Geometry: see drawing. Coordinates: mm, zero at the bounding-box minimum. A direction names the side the tool comes from. Round coordinates to 2 decimals unless told otherwise and drop trailing zeros. Loops run counter-clockwise (first coordinate to the right, second up) from the corner with the lowest first, then second, coordinate; pieces in that order, holes last. Notation, with made-up numbers: (51.25, 69.25) -> (86.25, 69.25) arc R31 cw to (86.25, 105.25) -> close; hole circle Ø9 at (84.25, 33.5). An arc over 180 degrees is marked (long way). Write item = value, one per line.
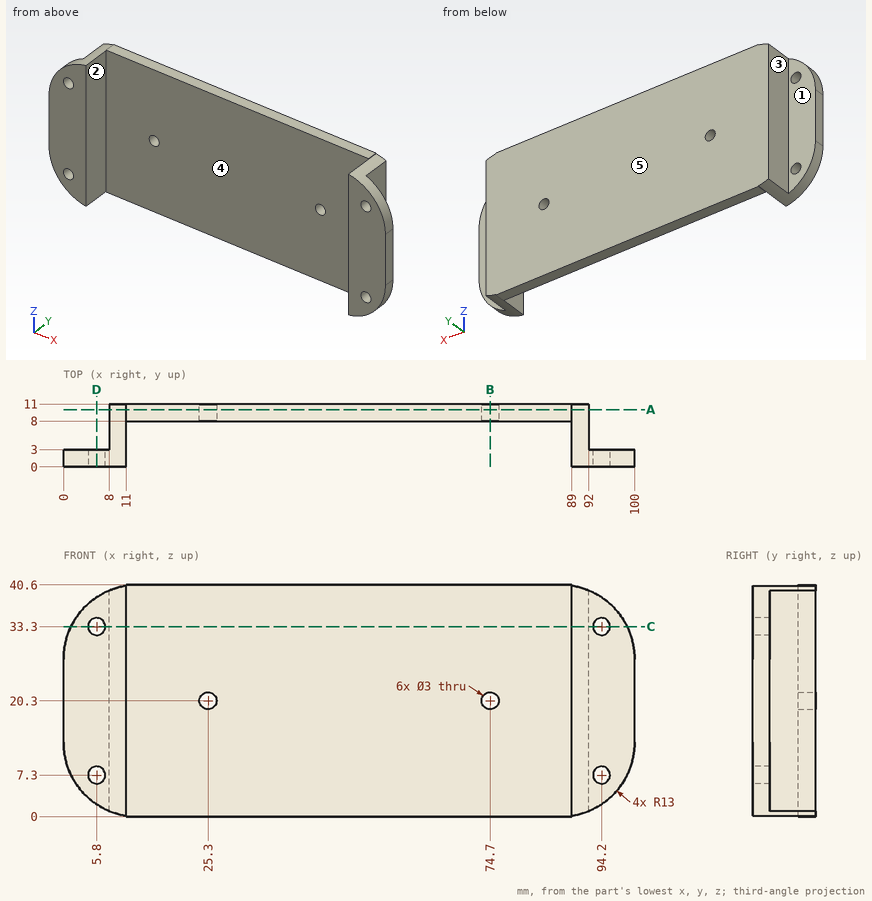
1. Section query C-C (z = 33.3). Return the cut outline in (x, y).
Evaluation:
outline = (1.32, 0) -> (4.3, 0) -> (4.3, 3) -> (1.32, 3) -> close; (7.3, 0) -> (11, 0) -> (11, 8) -> (89, 8) -> (89, 0) -> (92.7, 0) -> (92.7, 3) -> (92, 3) -> (92, 11) -> (8, 11) -> (8, 3) -> (7.3, 3) -> close; (95.7, 0) -> (98.68, 0) -> (98.68, 3) -> (95.7, 3) -> close
2. Section query B-B (x = 74.7). Return the cut outline in (y, z).
Evaluation:
outline = (8, 0) -> (11, 0) -> (11, 18.8) -> (8, 18.8) -> close; (8, 21.8) -> (11, 21.8) -> (11, 40.6) -> (8, 40.6) -> close
3. Contact query for flat-ended pins moving along their axis: pin 1 Ø4 at (x, z) = (5.5, 25.5) entering from +Y; pin 2 Ø2.5 at (y, z) = (6, 27.5) entering from +X; pin 3 Ø2 at (y, z) = (8.5, 13.5) entering from -X. Output: stop coordinate, or through.
Evaluation:
pin_1 = 3
pin_2 = 92
pin_3 = 8
4. Section query D-D (x = 5.8). Return the cut outline in (y, z).
Evaluation:
outline = (0, 2.18) -> (3, 2.18) -> (3, 5.8) -> (0, 5.8) -> close; (0, 8.8) -> (3, 8.8) -> (3, 31.8) -> (0, 31.8) -> close; (0, 34.8) -> (3, 34.8) -> (3, 38.42) -> (0, 38.42) -> close
5. Section query A-A (y = 10). Return the cut outline in (x, z).
Evaluation:
outline = (8, 1) arc R13 ccw to (11, 0.15) -> (11, 0) -> (89, 0) -> (89, 0.15) arc R13 ccw to (92, 1) -> (92, 39.6) arc R13 ccw to (89, 40.45) -> (89, 40.6) -> (11, 40.6) -> (11, 40.45) arc R13 ccw to (8, 39.6) -> close; hole circle Ø3 at (25.3, 20.3); hole circle Ø3 at (74.7, 20.3)
6. Line query: probe 1 along X at (y, z) = (9.8, 20.3); probe 2 along Z at (x, y) = (94.2, 2.2); probe 3 along X at (y, z) = (6.75, 28.5). Output: solid intervals per line, ascending. Write a range as from..to.
Evaluation:
probe_1 = 8..23.8, 26.8..73.2, 76.2..92
probe_2 = 2.18..5.8, 8.8..31.8, 34.8..38.42
probe_3 = 8..11, 89..92
7. Mould query, pull axis X, two halves, no side actions, for the marked faces 1, 2 and 3. Classes: released by +X, released by -X, zero draft, split by the parting line, or undercut.
Evaluation:
face_1 = zero draft
face_2 = undercut
face_3 = released by -X
8. Set-up query: the marked faces 4 and 5. Return all of +Z, -Z, +X, -X, +Y, -Y with unobstructed straight access to the full face (end or side cutting, diameter ignored); none if empty.
Evaluation:
face_4 = +Z, -Z, -Y
face_5 = +Z, -Z, +X, -X, +Y
